```python
from build123d import *

# Parameters (mm, degrees)
SKETCH_1_R               = 3
SKETCH_1_R_2             = 1
EXTRUDE_1_DEPTH          = 6
SKETCH_1_4_R             = 4
SKETCH_1_4_R_2           = 3
EXTRUDE_2_DEPTH          = 4
SKETCH_1_5_R             = 3
SKETCH_1_5_R_2           = 1
EXTRUDE_3_DEPTH          = 12
SKETCH_2_R               = 4
SKETCH_2_R_2             = 3
EXTRUDE_4_DEPTH          = 2
CUT_EXTRUDE_1_DEPTH      = 17.439282223
CUT_EXTRUDE_1_DEPTH_BACK = 17.439282223
SKETCH_3_W               = 6
SKETCH_3_H               = 12.2
EXTRUDE_7_DEPTH          = 2.5
CUT_EXTRUDE_2_DEPTH      = 1.1


with BuildPart() as part:
    # Sketch 1 → Extrude 1 (new, symmetric)
    with BuildSketch(Plane.XY):
        with Locations((6.5, 0)):
            Circle(SKETCH_1_R)
        with Locations((6.5, 0)):
            Circle(SKETCH_1_R_2, mode=Mode.SUBTRACT)
    extrude(amount=EXTRUDE_1_DEPTH, both=True)

    # Sketch 1_4 → Extrude 2 (add, symmetric)
    with BuildSketch(Plane.XY):
        with Locations((6.5, 0)):
            Circle(SKETCH_1_4_R)
        with Locations((6.5, 0)):
            Circle(SKETCH_1_4_R_2, mode=Mode.SUBTRACT)
    extrude(amount=EXTRUDE_2_DEPTH, both=True)



with BuildPart() as body_2:
    # Sketch 1_5 → Extrude 3 (new, symmetric)
    with BuildSketch(Plane.XY):
        with Locations((-6.5, 0)):
            Circle(SKETCH_1_5_R)
        with Locations((-6.5, 0)):
            Circle(SKETCH_1_5_R_2, mode=Mode.SUBTRACT)
    extrude(amount=EXTRUDE_3_DEPTH, both=True)

    # Sketch 2 → Extrude 4 (add, symmetric)
    with BuildSketch(Plane.XY.offset(9)):
        with Locations((-6.5, 0)):
            Circle(SKETCH_2_R)
        with Locations((-6.5, 0)):
            Circle(SKETCH_2_R_2, mode=Mode.SUBTRACT)
    extrude_4 = extrude(amount=EXTRUDE_4_DEPTH, both=True)

    # Mirror 1: Extrude 4 across plane
    add(extrude_4.mirror(Plane.XY))

    # Sketch 3 → Cut-Extrude 1 (cut, two sides: drawn at the far end of the back side and taken through both)
    with BuildSketch(Plane(origin=(0, 0, 0), x_dir=(1, 0, 0), z_dir=(0, 1, 0)).offset(-CUT_EXTRUDE_1_DEPTH_BACK)):
        with Locations((-6.5, 0)):
            Rectangle(SKETCH_3_W, SKETCH_3_H)
    extrude(amount=CUT_EXTRUDE_1_DEPTH + CUT_EXTRUDE_1_DEPTH_BACK, mode=Mode.SUBTRACT)


with BuildPart() as cut_extrude_1_piece_1:
    # of the separate pieces the step leaves, piece 1, a body of its own (cut_extrude_1_pieces)
    add(body_2.part.solids().sort_by_distance((-3.5, 0, -12))[0])


with BuildPart() as cut_extrude_1_piece_2:
    # of the separate pieces the step leaves, piece 2, a body of its own (cut_extrude_1_pieces)
    add(body_2.part.solids().sort_by_distance((-5.5, 0, 12))[0])


with BuildPart() as part_1:
    add(part.part)

    add(cut_extrude_1_piece_1.part)  # Extrude 7 merges Cut-Extrude 1 piece 1

    add(cut_extrude_1_piece_2.part)  # Extrude 7 merges Cut-Extrude 1 piece 2
    # Sketch 4 → Extrude 7 (add, symmetric)
    with BuildSketch(Plane(origin=(0, 0, 0), x_dir=(1, 0, 0), z_dir=(0, 1, 0))):
        Polygon((5.5, -6), (5.5, 6), (3.5, 6), (-3.5, 12), (-5.5, 12), (-5.5, 6.1), (-3.5, 6.1), (-2.5, 5), (-2.5, -5), (-3.5, -6.1), (-5.5, -6.1), (-5.5, -12), (-3.5, -12), (3.5, -6), align=None)
    extrude(amount=EXTRUDE_7_DEPTH, both=True)

    # Sketch 5 → Cut-Extrude 2 (cut, symmetric)
    with BuildSketch(Plane.XY):
        Polygon((-1.5, 2.5), (-2.5, -2.5), (-2.5, 2.5), align=None)
    extrude(amount=CUT_EXTRUDE_2_DEPTH, both=True, mode=Mode.SUBTRACT)


solid = part_1.part
```
For this review, take the finished solid that the model builds, in its own axes (mm). A direction names the side the tool comes from. Coordinates: 2 decimals unless noted, no trailing zeros. Order: outer loops, then holes, each group sorted by start corner. A loop starts at its lowest first (then second) coordinate and runs counter-clockwise, first axis right, second up. Notation, with made-up numbers: (85.25, -28.5) -> (91.25, -28.5) arc R8 cw to (91.25, -20.5) -> close; hole circle Ø11 at (8.25, 7.5). An arc over 180 degrees is marked (long way). Use CSV: the item, a comma, the result in double quotes. Start each with the question number.
Item 1: We need section D-D, the plane z = -0.75. Give the boundary of the cut face in (x, y), then the cut area to 3 significant figures.
Item 2: Wall thickness on probe 1 along Z at (x, y) = (-7.75, -1.25); probe 2 along Y at (x, z) = (6.5, 0); probe 3 along X at (y, z) = (0.25, -4.75): over which ranges is each line inside the solid? List them lowest first.
Item 3: Draft analysis for pull direction X (two halves, no side actions). For faces 4 (the face through (-7.3, -0.6, -9.1)), 5 (the face through (-2, 1, -1.1)), 6 (the face through (-10.5, 0.1, 9)), state which applies: pulls with the +X half, pulls with the -X half, needs draft (parallel to the pull), parting line crosses it, or undercut.
Item 4: For faces 1 (the face through (-10, 0, -7)), 2 (the face through (-5, 0, 6.1)), 3 (the face through (9.5, -0.1, 5)), list the 3-axis set-ups (+Z, -Z, +X, -X, +Y, -Y) from which the entire face can be reached by the end or side of a thin tool; tool diameter is ignored.
Item 5: We need section A-A, the plane x = 6.5. Give the boundary of the cut face in (y, z), then the cut area to 3 significant figures.
Item 6: We need section B-B, the plane x = -6.5. Give the number of separate pieces and of enclosed holes in the cut face, then the cut area to 3 significant figures.
Item 7: Insertion check: pin 1 (3 mm diameter, centred on y = 0, z = -4, fed in from -X); pin 2 (0.8 mm diameter, centred on x = -2, y = 1, fed in from +Z); pin 3 (1 mm diameter, centred on y = -3, z = -0.5, fed in from +X); pin 4 (2.5 mm diameter, centred on x = -6.5, y = 0, fed in from -Z). Each pin has a flat end and moves straight along its axis. Give the tip position at first contact, or say it passes through.
Derived:
1,outline,"(-2.5, -2.5) -> (3.38, -2.5) arc R4 ccw (long way) to (3.38, 2.5) -> (-1.5, 2.5) -> close; hole circle Ø2 at (6.5, 0)"
1,area,"71.0 mm^2"
2,probe 1,"z = -12 to -6.1, 6.1 to 12"
2,probe 2,"y = -4 to -1, 1 to 4"
2,probe 3,"x = -2.5 to 5.53, 7.47 to 9.49"
3,face 4,"undercut"
3,face 5,"needs draft"
3,face 6,"parting line crosses it"
4,face 1,"none"
4,face 2,"-X, +Y, -Y"
4,face 3,"+Z"
5,outline,"(-4, -4) -> (-3, -4) -> (-3, -6) -> (-1, -6) -> (-1, 6) -> (-3, 6) -> (-3, 4) -> (-4, 4) -> close; (1, -6) -> (3, -6) -> (3, -4) -> (4, -4) -> (4, 4) -> (3, 4) -> (3, 6) -> (1, 6) -> close"
5,area,"64.0 mm^2"
6,separate pieces,"4"
6,enclosed holes,"0"
6,area,"63.2 mm^2"
7,pin 1,"stops at x = -2.95"
7,pin 2,"stops at z = 11.06"
7,pin 3,"stops at x = 9.62"
7,pin 4,"stops at z = -12"
